```python
from build123d import *

# Parameters (mm, degrees)
SKETCH1_R           = 1.35
BOSS_EXTRUDE1_DEPTH = 4.275
SKETCH2_R           = 2.3
BOSS_EXTRUDE2_DEPTH = 1.15
SKETCH3_R           = 1.5
BOSS_EXTRUDE3_DEPTH = 1.15


with BuildPart() as part:
    # Sketch1 → Boss-Extrude1 (new, symmetric)
    with BuildSketch(Plane.XY):
        Circle(SKETCH1_R)
    extrude(amount=BOSS_EXTRUDE1_DEPTH, both=True)

    # Sketch2 → Boss-Extrude2 (add)
    with BuildSketch(Plane.XY.offset(4.275)):
        with Locations((0, 0.024044425)):
            Circle(SKETCH2_R)
    extrude(amount=BOSS_EXTRUDE2_DEPTH)

    # Sketch3 → Boss-Extrude3 (add)
    with BuildSketch(Plane(origin=(0, 0, -4.275), x_dir=(-1, 0, 0), z_dir=(0, 0, -1))):
        Circle(SKETCH3_R)
    extrude(amount=BOSS_EXTRUDE3_DEPTH)

    # Sketch4 → Cut-Revolve1 (revolve, cut)
    with BuildSketch(Plane(origin=(0, 0, 0), x_dir=(0, 0, -1), z_dir=(1, 0, 0)), mode=Mode.PRIVATE) as cut_revolve1_sk:
        Polygon((5.225, 0.2), (5.225, 0), (5.425, 0), (5.425, 1.5), (4.475, 1.5), align=None)
    revolve(cut_revolve1_sk.sketch.rotate(Axis((0, 0, -4.275), (0, 0, -1)), 180), axis=Axis((0, 0, -4.275), (0, 0, -1)), mode=Mode.SUBTRACT)


solid = part.part
```
The listing builds one solid part. Answer for the finished solid, in the listing's coordinates (mm). Give positions to 0.01 mm unless a question says otherwise; leave off trailing zeros. Order: outer loops, then holes, each group sorted by start corner. A loop starts at its lowest first (then second) coordinate and runs counter-clockwise, first axis right, second up. Notation, with made-up numbers: M 4,12.5 L 14,12.5 A4 ccw 14,16.5 Z; hole C 19.5,40 d4. An arc over 180 degrees is marked long. Put each result on its own line as item: value. Start each with the question number.
Item 1: The part is cut by section A-A, the plane x = 0. Determine the outline of the cut face in (y, z) (3 decimals), and give its area (4 significant figures).
Item 2: For a pull along Z with two mould halves and no side action, classify faces 1 (the face through (-0.29, -1.32, 0.06)), 2 (the face through (0, 0, 5.425)), 3 (the face through (-1.825, -1.375, 4.842)) as +Z half, -Z half, draft (parallel to the pull), parting line (faces both ways), or undercut.
Item 3: The part is cut by section D-D, the plane x = -1.75. Determine the outline of the cut face in (y, z) (3 decimals), and give its area (3 significant figures).
Item 4: Find the intervals of material crossed by line 1 along X through (y, z) = (0.1, 4.75); line 2 along Z through (x, y) = (-0.6, -1.5) (3 decimals); line 3 along Z through (x, y) = (-0.3, 1.35) (3 decimals), in increasing order.
Item 5: The part is cut by section C-C, the plane y = 2. Determine the outline of the cut face in (x, z) (3 decimals), and give its area (3 significant figures).
Item 6: The part is cut by section B-B, the plane z = 0.5. Determine the outline of the cut face in (x, y), and give its area (3 significant figures).
Item 7: Flat-ended cylindrical pins translate along their axes: P1, Ø1, axis at y = -1, z = 3, coming from the -X side; P2, Ø2, axis at x = 0.5, z = 3, coming from the +Y side; P3, Ø1.5, axis at x = -1, z = 1, coming from the -Y side. Find the tip coordinate at first contact, or state that the pin passes through.
Answer key:
1. outline: M -2.276,4.275 L -1.35,4.275 L -1.35,-4.275 L -1.5,-4.275 L -1.5,-4.475 L -0.2,-5.225 L 0.2,-5.225 L 1.5,-4.475 L 1.5,-4.275 L 1.35,-4.275 L 1.35,4.275 L 2.324,4.275 L 2.324,5.425 L -2.276,5.425 Z
1. area: 30.25 mm²
2. face 1: undercut
2. face 2: +Z half
2. face 3: draft
3. outline: M -1.468,4.275 L 1.517,4.275 L 1.517,5.425 L -1.468,5.425 Z
3. area: 3.43 mm²
4. line 1: x = -2.3 to 2.3
4. line 2: z = 4.275 to 5.425
4. line 3: z = -4.543 to -4.275, 4.275 to 5.425
5. outline: M -1.177,4.275 L 1.177,4.275 L 1.177,5.425 L -1.177,5.425 Z
5. area: 2.71 mm²
6. outline: C 0,0 d2.7
6. area: 5.73 mm²
7. P1: stops at x = -1.25
7. P2: stops at y = 1.35
7. P3: stops at y = -1.33
